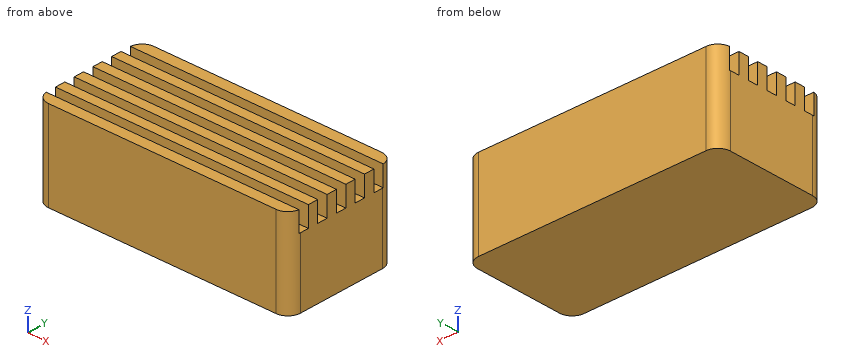
Autodesk Inventor part; units mm, degrees
ref_plane "YZ Plane" through (0, 0, 0) normal (1, 0, 0) x (0, 1, 0)
ref_plane "XZ Plane" through (0, 0, 0) normal (0, 1, 0) x (-1, 0, 0)
ref_plane "XY Plane" through (0, 0, 0) normal (0, 0, 1) x (1, 0, 0)
sketch "Sketch1" plane through (0, 0, 0) normal (0, 0, 1) x (1, 0, 0)
  line L0 (0, 0) -> (63.5, 0)
  line L1 (63.5, 0) -> (63.5, 28.575)
  line L2 (63.5, 28.575) -> (0, 28.575)
  line L3 (0, 28.575) -> (0, 0)
  dimension "d0" = 63.5
  dimension "d1" = 28.575
extrude "Extrusion1" add sketch "Sketch1" along normal blind 22.225
fillet "Fillet1" radius 3.175 4 edges at (63.5, 28.575, 11.1125) (63.5, 0, 11.1125) (0, 0, 11.1125) (0, 28.575, 11.1125)
sketch "Sketch2" plane through (0, 0, 22.225) normal (0, 0, 1) x (1, 0, 0)
  line L0 (63.5, 3.175) -> (63.5, 25.4)
  line L1 (0, 25.6349) -> (63.5, 25.6349)
  line L2 (63.5, 25.6349) -> (63.5, 23.0949)
  line L3 (63.5, 23.0949) -> (0, 23.0949)
  line L4 (0, 23.0949) -> (0, 25.6349)
  line L5 (0, 20.5549) -> (63.5, 20.5549)
  line L6 (63.5, 20.5549) -> (63.5, 18.0149)
  line L7 (63.5, 18.0149) -> (0, 18.0149)
  line L8 (0, 18.0149) -> (0, 20.5549)
  line L9 (0, 15.4749) -> (63.5, 15.4749)
  line L10 (63.5, 15.4749) -> (63.5, 12.9349)
  line L11 (63.5, 12.9349) -> (0, 12.9349)
  line L12 (0, 12.9349) -> (0, 15.4749)
  line L13 (0, 10.3949) -> (63.5, 10.3949)
  line L14 (63.5, 10.3949) -> (63.5, 7.8549)
  line L15 (63.5, 7.8549) -> (0, 7.8549)
  line L16 (0, 7.8549) -> (0, 10.3949)
  line L17 (0, 5.3149) -> (63.5, 5.3149)
  line L18 (63.5, 5.3149) -> (63.5, 2.7749)
  line L19 (63.5, 2.7749) -> (0, 2.7749)
  line L20 (0, 2.7749) -> (0, 5.3149)
  point P0 (0, 0)
  dimension "d5" = 2.54
  dimension "d8" = 5.08
extrude "Extrusion2" cut sketch "Sketch2" against normal blind 5.08
properties part number "Victor"
The model under review builds one solid part; all positions refer to its coordinate system, in mm. Give positions to 0.01 mm unless a question says otherwise; leave off trailing zeros. Write each loop counter-clockwise with the first axis right and the second up, starting at its lowest first coordinate (ties: lowest second). Pieces come first, ordered by that corner, then holes. Notation, with made-up numbers: (-11, 30.5) - (43, 30.5) arc R24 ccw to (43, 50.5) - close; hole circle Ø3 at (21, 71). An arc over 180 degrees is marked (long way). Answer in a Markdown table with one row per item. Add a question column.
1. We need section B-B on x = 57.5. Write out the cut boundary in (y, z) (3 decimals), then the cut area to 3 significant figures.
2. Wall thickness on line 1 along Y through (x, z) = (20.5, 19.75) (3 decimals); line 2 along Z through (x, y) = (57.5, 20.5) (3 decimals); line 3 along X through (y, z) = (25.75, 3): over which ranges is each line inside the solid? List them lowest first. Write a range as [from, to].
3. We need section A-A on z = 19.5. Write out the cut boundary in (x, y) (3 decimals), then the cut area to 3 significant figures.
4. Insertion check: P1, Ø0.8, axis at x = 19.5, y = 24.5, coming from the +Z side (3 decimals). The pin has a flat end and moves straight along its axis. Give the tip position at first contact, or say it passes through.
5. We need section C-C on y = 9.5. Write out the cut boundary in (x, z) (3 decimals).
Ans:
| question | item | result |
|---|---|---|
| 1 | outline | (0, 0) - (28.575, 0) - (28.575, 22.225) - (25.635, 22.225) - (25.635, 17.145) - (23.095, 17.145) - (23.095, 22.225) - (20.555, 22.225) - (20.555, 17.145) - (18.015, 17.145) - (18.015, 22.225) - (15.475, 22.225) - (15.475, 17.145) - (12.935, 17.145) - (12.935, 22.225) - (10.395, 22.225) - (10.395, 17.145) - (7.855, 17.145) - (7.855, 22.225) - (5.315, 22.225) - (5.315, 17.145) - (2.775, 17.145) - (2.775, 22.225) - (0, 22.225) - close |
| 1 | area | 571 mm^2 |
| 2 | line 1 | y = [0, 2.775], [5.315, 7.855], [10.395, 12.935], [15.475, 18.015], [20.555, 23.095], [25.635, 28.575] |
| 2 | line 2 | z = [0, 17.145] |
| 2 | line 3 | x = [0.02, 63.48] |
| 3 | outline | (0, 5.315) - (63.5, 5.315) - (63.5, 7.855) - (0, 7.855) - close; (0, 10.395) - (63.5, 10.395) - (63.5, 12.935) - (0, 12.935) - close; (0, 15.475) - (63.5, 15.475) - (63.5, 18.015) - (0, 18.015) - close; (0, 20.555) - (63.5, 20.555) - (63.5, 23.095) - (0, 23.095) - close; (0.009, 25.635) - (63.491, 25.635) arc R3.175 ccw to (60.325, 28.575) - (3.175, 28.575) arc R3.175 ccw to start; (0.025, 2.775) arc R3.175 ccw to (3.175, 0) - (60.325, 0) arc R3.175 ccw to (63.475, 2.775) - close |
| 3 | area | 999 mm^2 |
| 4 | P1 | stops at z = 17.145 |
| 5 | outline | (0, 0) - (63.5, 0) - (63.5, 17.145) - (0, 17.145) - close |
